```python
from build123d import *

# Parameters (mm, degrees)
F0_R      = 180
F1_DEPTH  = 10
F2_R      = 15
F2_R_2    = 7.5
F3_DEPTH  = 200
F5_R      = 180
F6_DEPTH  = 10
F7_R      = 15
F8_DEPTH  = 60
F10_R     = 15
F11_DEPTH = 60
F12_R     = 7.5
F13_DEPTH = 220


with BuildPart() as f1:
    # F0 (on Top) → F1 (new body)
    with BuildSketch(Plane.XY):
        Circle(F0_R)
    extrude(amount=F1_DEPTH)

    # F2 (on Top) → F3 (join)
    with BuildSketch(Plane.XY):
        Circle(F2_R)
        with Locations((0, 50)):
            Circle(F2_R_2)
        with Locations((-47.552826, 15.45085)):
            Circle(F2_R_2)
        with Locations((-29.389263, -40.45085)):
            Circle(F2_R_2)
        with Locations((29.389263, -40.45085)):
            Circle(F2_R_2)
        with Locations((47.552826, 15.45085)):
            Circle(F2_R_2)
    extrude(amount=F3_DEPTH)

    # F5 (on offset) → F6 (join)
    with BuildSketch(Plane.XY.offset(200)):
        Circle(F5_R)
    extrude(amount=F6_DEPTH)

    # F7 (on Top) → F8 (join)
    with BuildSketch(Plane.XY):
        Circle(F7_R)
    extrude(amount=-F8_DEPTH)

    # F10 (on offset) → F11 (join)
    with BuildSketch(Plane.XY.offset(210)):
        Circle(F10_R)
    extrude(amount=F11_DEPTH)

    # F12 (on Top) → F13 (cut)
    with BuildSketch(Plane.XY):
        with Locations((0, 75)):
            Circle(F12_R)
        with Locations((-68.905745, 24.937046)):
            Circle(F12_R)
        with Locations((-42.586093, -56.066516)):
            Circle(F12_R)
        with Locations((42.586093, -56.066516)):
            Circle(F12_R)
        with Locations((68.905745, 24.937046)):
            Circle(F12_R)
        with Locations((0, 102.548212)):
            Circle(F12_R)
        with Locations((-97.529145, 31.68914)):
            Circle(F12_R)
        with Locations((-60.276327, -82.963246)):
            Circle(F12_R)
        with Locations((60.276327, -82.963246)):
            Circle(F12_R)
        with Locations((97.529145, 31.68914)):
            Circle(F12_R)
    extrude(amount=F13_DEPTH, mode=Mode.SUBTRACT)


solid = f1.part
```
Source: CAD feature listing. Evaluate the final solid. Frame: model axes, mm. A direction names the side the tool comes from. Give positions to 0.01 mm unless a question says otherwise; leave off trailing zeros. Loops run counter-clockwise (first coordinate to the right, second up) from the corner with the lowest first, then second, coordinate; pieces in that order, holes last. Notation, with made-up numbers: (83, 33) -> (123, 33) arc R23 ccw to (123, 44) -> close; hole circle Ø4 at (18, 78.25). An arc over 180 degrees is marked (long way). Use a Markdown table: item, result. Add a question column.
(1) Section query B-B (y = 0). Output: boundary loops of the cut face in (x, z), then the cut area to 3 significant figures.
(2) First-contact query: pin 1 Ø9 at (x, y) = (-60.28, -82.96) entering from -Z; pin 2 Ø2 at (x, y) = (83.5, -119) entering from +Z; pin 3 Ø8 at (x, z) = (-51, 208.5) entering from +Y; pin 4 Ø12 at (x, y) = (24, -101.5) entering from -Z. Flat tips, straight axial feed; report the tip coordinate or a pass-through.
(3) Section query D-D (x = 0). Count the separate pieces of the cut face and the enclosed holes in it, then the cut area to 4 significant figures.
(4) Pull-direction query (Z, two-part tool) for faces 1 (the face through (-3, -37, 210)), 2 (the face through (52.784, -82.633, 204.93)), 3 (the face through (-3, -37, 10)); classes: +Z half, -Z half, draft (parallel to the pull), parting line (faces both ways), or undercut.
(5) Section query C-C (z = 67). Output: boundary loops of the cut face in (x, y).
(6) Ray query, line 1 (Y direction, x = 0, z = 207.25); line 2 (Z direction, x = -80, y = 88); line 3 (Y direction, x = 13, z = 234.5). Return the intervals inside material, ascending.
(7) Section query A-A (x = 113). Output: boundary loops of the cut face in (y, z).
(8) Access query for faces 4 (the face through (-0.976, 109.984, 4.93)), 5 (the face through (-14.985, 0.66, 239.58)), 6 (the face through (-55.046, 15.781, 103.67)). Directions: +Z, -Z, +X, -X, +Y, -Y. A direction counts if a zero-diameter tool reaches every point of the face in a straight line with its end or side. Return the directions, or none.
Checked values:
| question | item | result |
|---|---|---|
| 1 | outline | (-180, 0) -> (-15, 0) -> (-15, -60) -> (15, -60) -> (15, 0) -> (180, 0) -> (180, 10) -> (15, 10) -> (15, 200) -> (180, 200) -> (180, 210) -> (15, 210) -> (15, 270) -> (-15, 270) -> (-15, 210) -> (-180, 210) -> (-180, 200) -> (-15, 200) -> (-15, 10) -> (-180, 10) -> close |
| 1 | area | 16,500 mm^2 |
| 2 | pin 1 | through |
| 2 | pin 2 | z = 210 |
| 2 | pin 3 | y = 173.76 |
| 2 | pin 4 | z = 0 |
| 3 | separate pieces | 5 |
| 3 | enclosed holes | 1 |
| 3 | area | 18,750 mm^2 |
| 4 | face 1 | +Z half |
| 4 | face 2 | draft |
| 4 | face 3 | undercut |
| 5 | outline | circle Ø15 at (-47.55, 15.45); circle Ø15 at (-29.39, -40.45); circle Ø30 at (0, 0); circle Ø15 at (0, 50); circle Ø15 at (29.39, -40.45); circle Ø15 at (47.55, 15.45) |
| 6 | line 1 | -180 to 67.5, 82.5 to 95.05, 110.05 to 180 |
| 6 | line 2 | 0 to 10, 200 to 210 |
| 6 | line 3 | -7.48 to 7.48 |
| 7 | outline | (-140.11, 0) -> (140.11, 0) -> (140.11, 10) -> (-140.11, 10) -> close; (-140.11, 200) -> (140.11, 200) -> (140.11, 210) -> (-140.11, 210) -> close |
| 8 | face 4 | +Z, -Z |
| 8 | face 5 | +Z |
| 8 | face 6 | none |
